Part model, mm, in its own coordinate system. Coordinates: 2 decimals unless noted, no trailing zeros. Loops run counter-clockwise (first coordinate to the right, second up) from the corner with the lowest first, then second, coordinate; pieces in that order, holes last. Notation, with made-up numbers: M -29.75,-23.75 L 8.25,-23.75 A15 ccw 8.25,-19.75 Z; hole C 39,29.25 d9. An arc over 180 degrees is marked long. Use a Markdown table: item, result. Add a question column.
1) Band-saw the part on B-B (y = 12). List the corners of the cut face in (x, z), plus the area to 3 significant figures.
2) Wall check: probe 1 along Z at (x, y) = (-5, 12); probe 2 along X at (y, z) = (-2.5, 1); probe 3 along X at (y, z) = (13.5, 13.5). Give the ranges that are in metal, low to high. Write a range as from..to.
3) Band-saw the part on A-A (x = 19). List the corners of the cut face in (y, z).
from build123d import *

# Parameters (mm, degrees)
F0_W     = 60
F0_H     = 30
F1_DEPTH = 20
F2_SIZE  = 5
F3_SIZE  = 2


with BuildPart() as f1:
    # F0 (on Top) → F1 (new body)
    with BuildSketch(Plane.XY):
        Rectangle(F0_W, F0_H)
    extrude(amount=F1_DEPTH)

    # F2
    f2_edges = [f1.edges().sort_by_distance(p)[0] for p in [
        (0, -15, 20),
        (0, 15, 20),
        (0, -15, 0),
        (0, 15, 0),
    ]]
    chamfer(f2_edges, length=F2_SIZE)

    # F3
    f3_edges = [f1.edges().sort_by_distance(p)[0] for p in [
        (30, -15, 10),
        (30, -12.5, 2.5),
        (30, -12.5, 17.5),
        (30, 0, 0),
        (30, 0, 20),
        (30, 12.5, 2.5),
        (30, 12.5, 17.5),
        (30, 15, 10),
        (-30, 15, 10),
        (-30, 12.5, 2.5),
        (-30, 12.5, 17.5),
        (-30, 0, 0),
        (-30, 0, 20),
        (-30, -12.5, 2.5),
        (-30, -12.5, 17.5),
        (-30, -15, 10),
    ]]
    chamfer(f3_edges, length=F3_SIZE)


solid = f1.part
Entries:
| question | item | result |
|---|---|---|
| 1 | outline | M -30,4.83 L -28,2 L 28,2 L 30,4.83 L 30,15.17 L 28,18 L -28,18 L -30,15.17 Z |
| 1 | area | 949 mm2 |
| 2 | probe 1 | 2..18 |
| 2 | probe 2 | -29..29 |
| 2 | probe 3 | -29.5..29.5 |
| 3 | outline | M -15,5 L -10,0 L 10,0 L 15,5 L 15,15 L 10,20 L -10,20 L -15,15 Z |
